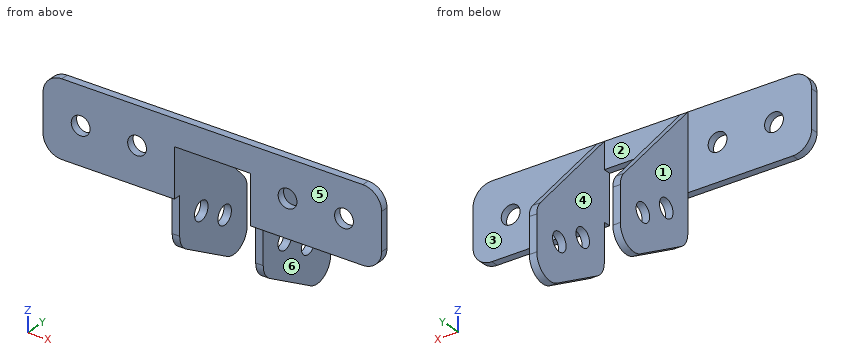
```python
from build123d import *

# Parameters (mm, degrees)
BOSS_EXTRUDE1_DEPTH = 2
SKETCH2_R           = 2.5
CUT_EXTRUDE1_DEPTH  = 47.14108798
BOSS_EXTRUDE2_DEPTH = 2
SKETCH4_R           = 2.5
CUT_EXTRUDE2_DEPTH  = 74.421360263
SKETCH5_R           = 2.5
BOSS_EXTRUDE3_DEPTH = 2
FILLET1_R           = 5
FILLET2_R           = 5


with BuildPart() as part:
    # Sketch1 → Boss-Extrude1 (new body)
    with BuildSketch(Plane(origin=(0, 0, 0), x_dir=(1, 0, 0), z_dir=(0, 1, 0))):
        Polygon((-10.1, 10), (-10.1, 0), (-10.1, -3), (10.1, -3), (10.1, 0), (10.1, 10), (45, 10), (45, -10), (-45, -10), (-45, 10), align=None)
    extrude(amount=BOSS_EXTRUDE1_DEPTH)

    # Sketch2 → Cut-Extrude1 (cut, through all)
    with BuildSketch(Plane(origin=(0, 2, 0), x_dir=(1, 0, 0), z_dir=(0, 1, 0))):
        with Locations(Location((-20, 0, 0), (0, 0, 270))):
            Circle(SKETCH2_R)
        with Locations(Location((-35, 0, 0), (0, 0, 270))):
            Circle(SKETCH2_R)
        with Locations(Location((20, 0, 0), (0, 0, 90))):
            Circle(SKETCH2_R)
        with Locations(Location((35, 0, 0), (0, 0, 90))):
            Circle(SKETCH2_R)
    extrude(amount=-CUT_EXTRUDE1_DEPTH, mode=Mode.SUBTRACT)

    # Sketch3 → Boss-Extrude2 (add)
    with BuildSketch(Plane.ZY.offset(-10.1)):
        Polygon((10, 2), (-17.43375673, 27), (-37.43375673, 27), (-23, 2), align=None)
    extrude(amount=-BOSS_EXTRUDE2_DEPTH)

    # Sketch4 → Cut-Extrude2 (cut, through all)
    with BuildSketch(Plane(origin=(12.1, 0, 0), x_dir=(0, 0, -1), z_dir=(1, 0, 0))):
        with Locations((22.46, 18.65)):
            Circle(SKETCH4_R)
        with Locations((17.46, 9.99)):
            Circle(SKETCH4_R)
    extrude(amount=-CUT_EXTRUDE2_DEPTH, mode=Mode.SUBTRACT)

    # Sketch5 → Boss-Extrude3 (add)
    with BuildSketch(Plane(origin=(-10.1, 0, 0), x_dir=(0, 0, -1), z_dir=(1, 0, 0))):
        Polygon((-10, 2), (17.43375673, 27), (37.43375673, 27), (23, 2), align=None)
        with Locations((22.46, 18.65)):
            Circle(SKETCH5_R, mode=Mode.SUBTRACT)
        with Locations((17.46, 9.99)):
            Circle(SKETCH5_R, mode=Mode.SUBTRACT)
    extrude(amount=-BOSS_EXTRUDE3_DEPTH)

    # Fillet1
    fillet1_edges = [part.edges().sort_by_distance(p)[0] for p in [
        (11.1, 2, -23),
        (11.1, 27, -37.43375673),
        (11.1, 27, -17.43375673),
        (-11.1, 2, -23),
        (-11.1, 27, -17.43375673),
        (-11.1, 27, -37.43375673),
    ]]
    fillet(fillet1_edges, radius=FILLET1_R)

    # Fillet2
    fillet2_edges = [part.edges().sort_by_distance(p)[0] for p in [
        (45, 1, 10),
        (-45, 1, 10),
        (-45, 1, -10),
        (45, 1, -10),
    ]]
    fillet(fillet2_edges, radius=FILLET2_R)


solid = part.part
```
CAD build for the part. Positions are in the model's coordinates, mm. Face numbers are marked on the shaded views. A direction names the side the tool comes from. Round coordinates to 2 decimals unless told otherwise and drop trailing zeros. Write each loop counter-clockwise with the first axis right and the second up, starting at its lowest first coordinate (ties: lowest second). Pieces come first, ordered by that corner, then holes.
Item 1: Band-saw the part on C-C on z = -22.46. Write the cut outline in (x, y), then the cut area to 3 significant figures.
Filled in:
outline: (-12.1, 2.58) - (-10.1, 2.58) - (-10.1, 16.15) - (-12.1, 16.15) - close; (-12.1, 21.15) - (-10.1, 21.15) - (-10.1, 27) - (-12.1, 27) - close; (10.1, 2.58) - (12.1, 2.58) - (12.1, 16.15) - (10.1, 16.15) - close; (10.1, 21.15) - (12.1, 21.15) - (12.1, 27) - (10.1, 27) - close
area: 77.7 mm2
Item 2: Drill centre lines: L1, parallel to X at y = 0.75, z = 0; L2, parallel to X at y = 14.5, z = -25; L3, parallel to Y at x = -11.1, z = -17.46. Where is each one in solid material? Low to high.
Filled in:
L1: x = -45 to -37.5, -32.5 to -22.5, -17.5 to -10.1, 10.1 to 17.5, 22.5 to 32.5, 37.5 to 45
L2: x = -12.1 to -10.1, 10.1 to 12.1
L3: y = 2 to 7.49, 12.49 to 26.62
Item 3: Band-saw the part on B-B on y = 9.99. Write the cut outline in (x, z), then the cut area to 3 significant figures.
Filled in:
outline: (-12.1, -27.61) - (-10.1, -27.61) - (-10.1, -19.96) - (-12.1, -19.96) - close; (-12.1, -14.96) - (-10.1, -14.96) - (-10.1, 1.23) - (-12.1, 1.23) - close; (10.1, -27.61) - (12.1, -27.61) - (12.1, -19.96) - (10.1, -19.96) - close; (10.1, -14.96) - (12.1, -14.96) - (12.1, 1.23) - (10.1, 1.23) - close
area: 95.4 mm2
Item 4: Band-saw the part on D-D on x = -16. Write the cut outline in (y, z).
Filled in:
outline: (0, -10) - (2, -10) - (2, 10) - (0, 10) - close
Item 5: Band-saw the part on A-A on x = -35. Write the cut outline in (y, z), then the cut area to 3 significant figures.
Filled in:
outline: (0, -10) - (2, -10) - (2, -2.5) - (0, -2.5) - close; (0, 2.5) - (2, 2.5) - (2, 10) - (0, 10) - close
area: 30.0 mm2
Item 6: Tool access for the marked faces 1, 2 and 3: list every direction of +Z, -Z, +X, -X, +Y, -Y with a clear straight run to the whole face (end or side of a thin tool).
Filled in:
face 1: +Z, -Z, -X, +Y
face 2: +Z, -Z, +Y
face 3: +Z, -Z, +X, +Y
Item 7: Drop flat-ended pins along their axis: pin 1 Ø12 at (y, z) = (23.5, -14) entering from +X; pin 2 Ø0.6 at (x, z) = (-11, -13) entering from -Y; pin 3 Ø2 at (x, z) = (-33, -6.5) entering from -Y; pin 4 Ø6.5 at (y, z) = (18.65, -22.46) entering from -X. Give the stop position or say it passes through.
Filled in:
pin 1: stops at x = 12.1
pin 2: stops at y = 2
pin 3: stops at y = 0
pin 4: stops at x = -12.1
Item 8: Mould opens along X. For the marked faces 4, 5 and 6 say: released by +X, released by -X, zero draft, split by the parting line, or undercut.
Filled in:
face 4: undercut
face 5: zero draft
face 6: released by +X
